Here's the drawing with two shaded views (mm, measured from the low corner). I have some questions. A direction names the side the tool comes from. Coordinates: 2 decimals unless noted, no trailing zeros. Write each loop counter-clockwise with the first axis right and the second up, starting at its lowest first coordinate (ties: lowest second). Pieces come first, ordered by that corner, then holes. Notation, with made-up numbers: M 80,2.5 L 136,2.5 A27 ccw 136,39.5 Z; hole C 38,36.25 d2. An arc over 180 degrees is marked long. Answer as CSV lines item,"result". Start each with the question number.
Item 1: Suppose I cut it at B-B, the plane x = 35.56. Write out the boundary of the cut face in (y, z), and give its area (3 significant figures).
Item 2: We'd pull the mould along X, two halves only. Please class the marked faces 4, 5, 6 and 7: +X half, -X half, draft (parallel to the pull), parting line (faces both ways), or undercut.
Item 3: I'm going to push flat-ended pins straight in: P1, Ø1.5, axis at x = 25, z = 9.5, coming from the +Y side; P2, Ø3, axis at x = 37, y = 34.5, coming from the -Z side; P3, Ø1, axis at x = 10.5, z = 8.5, coming from the -Y side. Where does each tip first touch, or does it pass through?
Item 4: Suppose I cut it at D-D, the plane z = 11.43. Write out the boundary of the cut face in (x, y).
Item 5: Suppose I cut it at C-C, the plane y = 34.29. Write out the boundary of the cut face in (x, z).
Item 6: Suppose I cut it at A-A, the plane y = 24.5. Write out the boundary of the cut face in (x, z).
Item 7: On a 3-axis mill with a long thin cutter (end or side, diameter ignored), from which of +Z, -Z, +X, -X, +Y, -Y can I reach the whole of each face in a straight line? I mean the marked faces 1, 2 and 3. Say none if no direction works.
Item 8: If I drill on line 1 along X through (y, z) = (12.5, 13.5); line 2 along Z through (x, y) = (41, 37); line 3 along Y through (x, z) = (8.5, 7), over which ranges is the centre line in solid material (lowest first)? Write a range as [from, to].
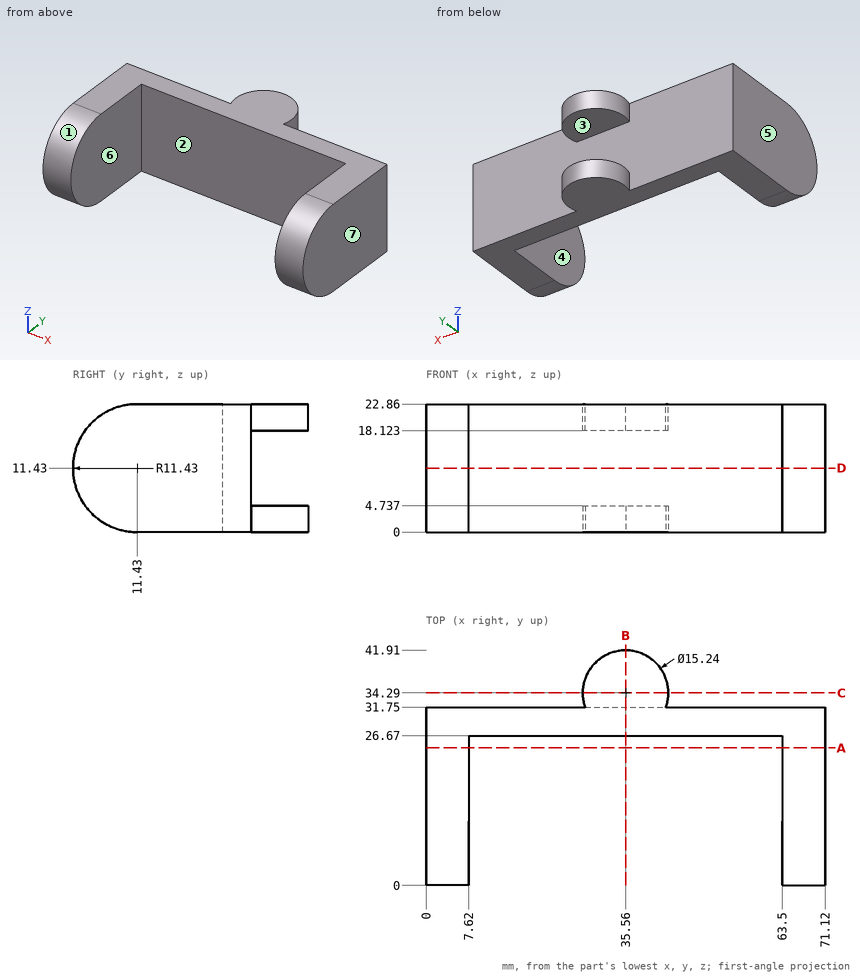
Ans:
1,outline,"M 26.67,0 L 41.91,0 L 41.91,4.74 L 31.75,4.74 L 31.75,18.12 L 41.91,18.12 L 41.91,22.86 L 26.67,22.86 Z"
1,area,"212 mm^2"
2,face 4,"undercut"
2,face 5,"-X half"
2,face 6,"undercut"
2,face 7,"+X half"
3,P1,"stops at y = 31.75"
3,P2,"stops at z = 0"
3,P3,"stops at y = 26.67"
4,outline,"M 0,0 L 7.62,0 L 7.62,26.67 L 63.5,26.67 L 63.5,0 L 71.12,0 L 71.12,31.75 L 0,31.75 Z"
5,outline,"M 27.94,0 L 43.18,0 L 43.18,4.74 L 27.94,4.74 Z; M 27.94,18.12 L 43.18,18.12 L 43.18,22.86 L 27.94,22.86 Z"
6,outline,"M 0,0 L 7.62,0 L 7.62,22.86 L 0,22.86 Z; M 63.5,0 L 71.12,0 L 71.12,22.86 L 63.5,22.86 Z"
7,face 1,"+X, -X, -Y"
7,face 2,"+Z, -Z, -Y"
7,face 3,"+X, -X, +Y"
8,line 1,"x = [0, 7.62], [63.5, 71.12]"
8,line 2,"z = [0, 4.74], [18.12, 22.86]"
8,line 3,"y = [26.67, 31.75]"
